Could you check a few things on this model? Use its own coordinates, in mm. A direction names the side the tool comes from. Give positions to 0.01 mm unless a question says otherwise; leave off trailing zeros. Order: outer loops, then holes, each group sorted by start corner. A loop starts at its lowest first (then second) coordinate and runs counter-clockwise, first axis right, second up. Notation, with made-up numbers: (49.5, 89.5) - (73.5, 89.5) arc R24 cw to (73.5, 116.5) - close; hole circle Ø8 at (65, 38). An arc over 180 degrees is marked (long way). One line per question, with ' | ' between items. Start each with the question number.
1. If we mould it in two halves opening along Z, with no side actions, what happens to faces 3 (the cylindrical face through (-71.672, 1.479, -10.924)), 4 (the cylindrical face through (-15.6, 1.5, -70.8)), 5 (the cylindrical face through (57.61, 1.52, 14.75)), 6 (the cylindrical face through (32.544, 1.479, 64.492))? For each: released by +Z, released by -Z, zero draft, split by the parting line, or undercut.
2. For P1, Ø3, axis at x = -55.72, z = -23.1, coming from the +Y side; P2, Ø1.5, axis at y = 0.5, z = -56.5, coming from the +X side; P3, Ø0.9, axis at y = 1.5, z = 57.5, coming from the +X side; P4, Ø1.5, axis at y = 2, z = -49.5, coming from the +X side, each with a flat end and sliding along its axis, tell me the tip position at first contact or that it passes through.
3. I need wall thicknesses on probe 1 along X at (y, z) = (1, 44); probe 2 along X at (y, z) = (0.75, 0) (3 decimals); probe 3 along X at (y, z) = (2.35, -23.1). Which ranges of each line are inside material? Lowest first, please. Write a range as from..to.
4. Which directions (+Z, -Z, +X, -X, +Y, -Y) give clear straight access to the entire face, cutting with the end or side of a thin tool? Please do faces 1 (the flat face through (42, 2, -15)), 2 (the conical face through (35.934, 1.875, -46.249)).
5. Imagine slicing it at C-C (z = -38). Please give me the cut outline in (x, y), and give its area (3 significant figures).
6. Imagine slicing it at B-B (y = 2.5). Give the number of separate pieces and of enclosed holes in the cut face, and give its area (3 significant figures).
7. Imagine slicing it at A-A (z = 39). Please give me the cut outline in (x, y), and give its area (3 significant figures).
```python
from build123d import *
from OCP.BRepFilletAPI import BRepFilletAPI_MakeChamfer

# Parameters (mm, degrees)
SKETCH1_W           = 3.175
SKETCH1_H           = 12.7
BOSS_EXTRUDE1_DEPTH = 3
SKETCH2_R           = 1.5
CUT_EXTRUDE1_DEPTH  = 103.574363269
CHAMFER1_SIZE       = 1.5
CHAMFER1_SIZE2      = 1.303930107
CUT_EXTRUDE2_DEPTH  = 103.574363269
SKETCH4_W           = 20
SKETCH4_H           = 1.7
CUT_EXTRUDE3_DEPTH  = 103.574363269
SKETCH5_R           = 5
CUT_EXTRUDE4_DEPTH  = 103.085748271
SKETCH6_R           = 1.8415
CUT_EXTRUDE5_DEPTH  = 103.085748271
SKETCH8_R           = 1.905
SKETCH8_W           = 10
SKETCH8_H           = 30
CUT_EXTRUDE7_DEPTH  = 103.085748271
CHAMFER2_SIZE       = 2
CHAMFER2_SIZE_2     = 1.738573476


with BuildPart() as part:
    # Sketch1 → Boss-Extrude1 (new body)
    with BuildSketch(Plane(origin=(0, 0, 0), x_dir=(1, 0, 0), z_dir=(0, 1, 0))):
        with BuildLine():
            Line((30.029977361, -64.812867647), (-30.029977361, -64.812867647))
            ThreePointArc((-30.029977361, -64.812867647), (-32.509837414, -64.500503794), (-34.834773739, -63.582926471))
            ThreePointArc((-34.834773739, -63.582926471), (0, 72.5), (34.834773739, -63.582926471))
            ThreePointArc((34.834773739, -63.582926471), (32.509837414, -64.500503794), (30.029977361, -64.812867647))
        make_face()
        with Locations((-66.9125, 0)):
            Rectangle(SKETCH1_W, SKETCH1_H, mode=Mode.SUBTRACT)
    extrude(amount=BOSS_EXTRUDE1_DEPTH)

    # Sketch2 → Cut-Extrude1 (cut, through all)
    with BuildSketch(Plane(origin=(0, 3, 0), x_dir=(1, 0, 0), z_dir=(0, 1, 0))):
        with Locations(Location((-30.5, 44, 0), (0, 0, 270))):
            Circle(SKETCH2_R)
        with Locations(Location((30.5, 44, 0), (0, 0, 270))):
            Circle(SKETCH2_R)
        with Locations(Location((30.5, 0, 0), (0, 0, 270))):
            Circle(SKETCH2_R)
        with Locations(Location((30.5, -44, 0), (0, 0, 270))):
            Circle(SKETCH2_R)
        with Locations(Location((-30.5, -44, 0), (0, 0, 270))):
            Circle(SKETCH2_R)
        with Locations(Location((-30.5, 0, 0), (0, 0, 270))):
            Circle(SKETCH2_R)
    extrude(amount=-CUT_EXTRUDE1_DEPTH, mode=Mode.SUBTRACT)

    # Chamfer1: one chamfer whose edges measure the first distance from different faces: ONE call of the kernel's chamfer builder (chamfer() names one face for all edges)
    chamfer1_edges_1 = [part.edges().sort_by_distance(p)[0] for p in [
        (-30.5, 3, -45.5),
    ]]
    chamfer1_side_1 = [part.faces().sort_by_distance(p)[0] for p in [
        (-30.5, 1.5, -45.5),
    ]]
    chamfer1_edges_2 = [part.edges().sort_by_distance(p)[0] for p in [
        (-30.5, 3, -1.5),
    ]]
    chamfer1_side_2 = [part.faces().sort_by_distance(p)[0] for p in [
        (-30.5, 1.5, -1.5),
    ]]
    chamfer1_edges_3 = [part.edges().sort_by_distance(p)[0] for p in [
        (-30.5, 3, 42.5),
    ]]
    chamfer1_side_3 = [part.faces().sort_by_distance(p)[0] for p in [
        (-30.5, 1.5, 42.5),
    ]]
    chamfer1_edges_4 = [part.edges().sort_by_distance(p)[0] for p in [
        (30.5, 3, 42.5),
    ]]
    chamfer1_side_4 = [part.faces().sort_by_distance(p)[0] for p in [
        (30.5, 1.5, 42.5),
    ]]
    chamfer1_edges_5 = [part.edges().sort_by_distance(p)[0] for p in [
        (30.5, 3, -1.5),
    ]]
    chamfer1_side_5 = [part.faces().sort_by_distance(p)[0] for p in [
        (30.5, 1.5, -1.5),
    ]]
    chamfer1_edges_6 = [part.edges().sort_by_distance(p)[0] for p in [
        (30.5, 3, -45.5),
    ]]
    chamfer1_side_6 = [part.faces().sort_by_distance(p)[0] for p in [
        (30.5, 1.5, -45.5),
    ]]
    chamfer1 = BRepFilletAPI_MakeChamfer(part.part.solid().wrapped)
    for e in chamfer1_edges_1:
        chamfer1.Add(CHAMFER1_SIZE, CHAMFER1_SIZE2, e.wrapped, chamfer1_side_1[0].wrapped)  # the first distance lies on this face
    for e in chamfer1_edges_2:
        chamfer1.Add(CHAMFER1_SIZE, CHAMFER1_SIZE2, e.wrapped, chamfer1_side_2[0].wrapped)  # the first distance lies on this face
    for e in chamfer1_edges_3:
        chamfer1.Add(CHAMFER1_SIZE, CHAMFER1_SIZE2, e.wrapped, chamfer1_side_3[0].wrapped)  # the first distance lies on this face
    for e in chamfer1_edges_4:
        chamfer1.Add(CHAMFER1_SIZE, CHAMFER1_SIZE2, e.wrapped, chamfer1_side_4[0].wrapped)  # the first distance lies on this face
    for e in chamfer1_edges_5:
        chamfer1.Add(CHAMFER1_SIZE, CHAMFER1_SIZE2, e.wrapped, chamfer1_side_5[0].wrapped)  # the first distance lies on this face
    for e in chamfer1_edges_6:
        chamfer1.Add(CHAMFER1_SIZE, CHAMFER1_SIZE2, e.wrapped, chamfer1_side_6[0].wrapped)  # the first distance lies on this face
    add(Compound.cast(chamfer1.Shape()), mode=Mode.REPLACE)

    # Sketch3 → Cut-Extrude2 (cut, through all)
    with BuildSketch(Plane(origin=(0, 3, 0), x_dir=(1, 0, 0), z_dir=(0, 1, 0))):
        Polygon((1.35, -61.812867647), (3.1, -61.812867647), (3.1, -59.612867647), (1.35, -59.612867647), (1.35, -55.812867647), (-1.35, -55.812867647), (-1.35, -59.612867647), (-3.1, -59.612867647), (-3.1, -61.812867647), (-1.35, -61.812867647), (-1.35, -64.812867647), (1.35, -64.812867647), align=None)
    extrude(amount=-CUT_EXTRUDE2_DEPTH, mode=Mode.SUBTRACT)

    # Sketch4 → Cut-Extrude3 (cut, through all)
    with BuildSketch(Plane(origin=(0, 3, 0), x_dir=(1, 0, 0), z_dir=(0, 1, 0))):
        with Locations((0, 70.957033082)):
            Rectangle(SKETCH4_W, SKETCH4_H)
    extrude(amount=-CUT_EXTRUDE3_DEPTH, mode=Mode.SUBTRACT)


with BuildPart() as body_2:
    # of the pieces the cut leaves, the one that is kept (cut_extrude3_keep)
    add(part.part.solids().sort_by_distance((-30.029977361, 3, 64.812867647))[0])

    # Sketch5 → Cut-Extrude4 (cut, through all)
    with BuildSketch(Plane(origin=(0, 3, 0), x_dir=(1, 0, 0), z_dir=(0, 1, 0))):
        with Locations(Location((0, 65, 0), (0, 0, 270))):
            Circle(SKETCH5_R)
        with Locations(Location((30, -57, 0), (0, 0, 90))):
            Circle(SKETCH5_R)
        with Locations(Location((-30, -57, 0), (0, 0, 270))):
            Circle(SKETCH5_R)
    extrude(amount=-CUT_EXTRUDE4_DEPTH, mode=Mode.SUBTRACT)

    # Sketch6 → Cut-Extrude5 (cut, through all)
    with BuildSketch(Plane(origin=(0, 3, 0), x_dir=(1, 0, 0), z_dir=(0, 1, 0))):
        with Locations(Location((-34.29, 47.297033082, 0), (0, 0, 270))):
            Circle(SKETCH6_R)
        with Locations(Location((-34.29, 4.117033082, 0), (0, 0, 270))):
            Circle(SKETCH6_R)
        with Locations(Location((34.29, 4.117033082, 0), (0, 0, 270))):
            Circle(SKETCH6_R)
        with Locations(Location((34.29, 47.297033082, 0), (0, 0, 270))):
            Circle(SKETCH6_R)
    extrude(amount=-CUT_EXTRUDE5_DEPTH, mode=Mode.SUBTRACT)

    # Sketch8 → Cut-Extrude7 (cut, through all)
    with BuildSketch(Plane(origin=(0, 3, 0), x_dir=(1, 0, 0), z_dir=(0, 1, 0))):
        with Locations(Location((55.721466806, -15, 0), (0, 0, 270))):
            Circle(SKETCH8_R)
        with Locations(Location((55.721466806, 23.1, 0), (0, 0, 270))):
            Circle(SKETCH8_R)
        with Locations(Location((19.05, -52.812867647, 0), (0, 0, 270))):
            Circle(SKETCH8_R)
        with Locations(Location((-19.05, -52.812867647, 0), (0, 0, 270))):
            Circle(SKETCH8_R)
        with Locations(Location((-55.721466806, 23.1, 0), (0, 0, 270))):
            Circle(SKETCH8_R)
        with Locations(Location((-55.721466806, -15, 0), (0, 0, 270))):
            Circle(SKETCH8_R)
        with Locations((-42.5, 0)):
            Rectangle(SKETCH8_W, SKETCH8_H)
        with Locations((42.5, 0)):
            Rectangle(SKETCH8_W, SKETCH8_H)
        with BuildLine():
            Line((-23.730146131, 68.506424258), (-22.894827642, 65.923344486))
            ThreePointArc((-22.894827642, 65.923344486), (-18.461538462, 57.089154816), (-20.040369901, 66.846421409))
            Line((-20.040369901, 66.846421409), (-20.87568839, 69.429501181))
            ThreePointArc((-20.87568839, 69.429501181), (-22.764455722, 70.39519159), (-23.730146131, 68.506424258))
        make_face()
        with BuildLine():
            Line((20.040369901, 66.846421409), (20.87568839, 69.429501181))
            ThreePointArc((20.87568839, 69.429501181), (22.764455722, 70.39519159), (23.730146131, 68.506424258))
            Line((23.730146131, 68.506424258), (22.894827642, 65.923344486))
            ThreePointArc((22.894827642, 65.923344486), (18.461538462, 57.089154816), (20.040369901, 66.846421409))
        make_face()
        with BuildLine():
            ThreePointArc((39.925125077, -60.516397675), (40.640278394, -56.379231744), (44.791355024, -57.008635443))
            ThreePointArc((44.791355024, -57.008635443), (42.394535015, -58.812867647), (39.925125077, -60.516397675))
        make_face()
        with BuildLine():
            ThreePointArc((-39.925125077, -60.516397675), (-40.640278394, -56.379231744), (-44.791355024, -57.008635443))
            ThreePointArc((-44.791355024, -57.008635443), (-42.394535015, -58.812867647), (-39.925125077, -60.516397675))
        make_face()
    extrude(amount=-CUT_EXTRUDE7_DEPTH, mode=Mode.SUBTRACT)

    # Chamfer2
    # the kernel refuses this chamfer: 2, 1.738573476 mm, written as the material it takes off along each edge
    with BuildSketch(Plane(origin=(-19.05, 0, 52.812867647), x_dir=(0, 0, 1), z_dir=(-1, 0, 0))) as chamfer2_piece_1:
        Polygon((1.905, CHAMFER2_SIZE), (1.905 + CHAMFER2_SIZE_2, 0), (1.905, 0), align=None)
    revolve(axis=Axis((-19.05, 0, 52.812867647), (0, 1, 0)), mode=Mode.SUBTRACT)
    with BuildSketch(Plane(origin=(19.05, 0, 52.812867647), x_dir=(0, 0, 1), z_dir=(-1, 0, 0))) as chamfer2_piece_2:
        Polygon((1.905, CHAMFER2_SIZE), (1.905 + CHAMFER2_SIZE_2, 0), (1.905, 0), align=None)
    revolve(axis=Axis((19.05, 0, 52.812867647), (0, 1, 0)), mode=Mode.SUBTRACT)
    with BuildSketch(Plane(origin=(-34.29, 0, -47.297033082), x_dir=(0, 0, 1), z_dir=(-1, 0, 0))) as chamfer2_piece_3:
        Polygon((1.8415, CHAMFER2_SIZE_2), (1.8415 + CHAMFER2_SIZE, 0), (1.8415, 0), align=None)
    revolve(axis=Axis((-34.29, 0, -47.297033082), (0, 1, 0)), mode=Mode.SUBTRACT)
    with BuildSketch(Plane(origin=(-34.29, 0, -4.117033082), x_dir=(0, 0, 1), z_dir=(-1, 0, 0))) as chamfer2_piece_4:
        Polygon((1.8415, CHAMFER2_SIZE), (1.8415 + CHAMFER2_SIZE_2, 0), (1.8415, 0), align=None)
    revolve(axis=Axis((-34.29, 0, -4.117033082), (0, 1, 0)), mode=Mode.SUBTRACT)
    with BuildSketch(Plane(origin=(34.29, 0, -4.117033082), x_dir=(0, 0, 1), z_dir=(-1, 0, 0))) as chamfer2_piece_5:
        Polygon((1.8415, CHAMFER2_SIZE), (1.8415 + CHAMFER2_SIZE_2, 0), (1.8415, 0), align=None)
    revolve(axis=Axis((34.29, 0, -4.117033082), (0, 1, 0)), mode=Mode.SUBTRACT)
    with BuildSketch(Plane(origin=(34.29, 0, -47.297033082), x_dir=(0, 0, 1), z_dir=(-1, 0, 0))) as chamfer2_piece_6:
        Polygon((1.8415, CHAMFER2_SIZE), (1.8415 + CHAMFER2_SIZE_2, 0), (1.8415, 0), align=None)
    revolve(axis=Axis((34.29, 0, -47.297033082), (0, 1, 0)), mode=Mode.SUBTRACT)


solid = body_2.part
```
Results found:
1) face 3: split by the parting line | face 4: released by -Z | face 5: undercut | face 6: released by +Z
2) P1: passes through | P2: stops at x = 46.35 | P3: stops at x = 39.97 | P4: stops at x = 53.66
3) probe 1: x = -57.62..-32, -29..29, 32..57.62 | probe 2: x = -72.5..-68.5, -65.325..-47.5, -37.5..-32, -29..29, 32..37.5, 47.5..72.5 | probe 3: x = -68.72..-57.63, -53.82..53.82, 57.63..68.72
4) face 1: +Y, -Y | face 2: -Y
5) outline: (-61.74, 0) - (61.74, 0) - (61.74, 3) - (-61.74, 3) - close | area: 370 mm2
6) separate pieces: 1 | enclosed holes: 22 | area: 14,800 mm2
7) outline: (-61.12, 0) - (61.12, 0) - (61.12, 3) - (-61.12, 3) - close | area: 367 mm2
